Geometry check sheet. Reference: the model listing, model coordinates, mm. A direction names the side the tool comes from. Round coordinates to 2 decimals unless told otherwise and drop trailing zeros. Write each loop counter-clockwise with the first axis right and the second up, starting at its lowest first coordinate (ties: lowest second). Pieces come first, ordered by that corner, then holes.
Item 1: Cross-section at C-C (y = 18). Enter the section's corners in (x, z), then the cut area to 3 significant figures.
Item 2: Access from +Z, -Z, +X, -X, +Y, -Y to the whole of each face (thin tool, end or side, straight path). Record for faces 5 (the face through (7.612, 15, -63)), 6 (the face through (20, 6, -109)), 7 (the face through (47.99, 6.55, -21.06)), 8 (the face through (34.094, 10, -63)).
Item 3: Cross-section at A-A (x = 18). Enter the section's corners in (y, z).
Item 4: Cross-section at B-B (z = -104). Enter the section's corners in (x, y).
Item 5: Depth check by flat-ended pin: P1, Ø6, axis at x = 30.5, z = -69, coming from the +Y side; P2, Ø10, axis at y = 15, z = -103, coming from the +X side; P3, Ø1.5, axis at x = 34, y = 8.5, coming from the +Z side; P4, Ø1.7, axis at y = 10, z = -20, coming from the -X side. Enter the tip coordinate at first touch or a pass-through.
Item 6: Draft check along Z on faces 1 (the face through (40, 10, -59)), 2 (the face through (-2.96, 7.24, -98.07)), 3 (the face through (4.34, 9.86, -54.587)), 4 (the face through (48, 10, -30)). Enter one of: pulls with the +Z half, pulls with the -Z half, needs draft (parallel to the pull), parting line crosses it, or undercut.
Item 7: Cross-section at D-D (x = 36.5). Enter the section's corners in (y, z).
Item 8: Scan lines: probe 1 along Z at (x, y) = (26.5, 14.75); probe 2 along Y at (x, z) = (15, -109); probe 3 along X at (y, z) = (14, -20.5). Record each from-to range of solid material in increasing order.
from build123d import *

# Parameters (mm, degrees)
AUFSATZ_LINEAR_AUSTRAGEN1_DEPTH      = 20
SCHNITT_LINEAR_AUSTRAGEN1_DEPTH      = 53.24
SKIZZE3_R                            = 3.1
SCHNITT_LINEAR_AUSTRAGEN2_DEPTH      = 53.24
SCHNITT_LINEAR_AUSTRAGEN3_DEPTH      = 2
SKIZZE5_R                            = 0.75
SCHNITT_LINEAR_AUSTRAGEN4_DEPTH      = 2
AUFSATZ_LINEAR_AUSTRAGEN2_DEPTH      = 20
SKIZZE7_W                            = 7.611739691
SKIZZE7_H                            = 51.890970688
AUFSATZ_LINEAR_AUSTRAGEN3_DEPTH      = 20
SKIZZE8_W                            = 11.248625368
SKIZZE8_H                            = 20
AUFSATZ_LINEAR_AUSTRAGEN4_DEPTH      = 26.48
SCHNITT_LINEAR_AUSTRAGEN5_DEPTH      = 26.48
SCHNITT_LINEAR_AUSTRAGEN6_DEPTH      = 6
SCHNITT_LINEAR_AUSTRAGEN6_DEPTH_BACK = 26.48
SKIZZE10_R                           = 1.75
SKIZZE11_R                           = 3
AUFSATZ_LINEAR_AUSTRAGEN5_DEPTH      = 6


with BuildPart() as part:
    # Skizze1 → Aufsatz-Linear austragen1 (new body)
    with BuildSketch(Plane(origin=(0, 0, 0), x_dir=(1, 0, 0), z_dir=(0, 1, 0))):
        with BuildLine():
            Line((0, 59), (0, 0))
            Line((0, 0), (3, 0))
            Line((3, 0), (3, 51.3))
            ThreePointArc((3, 51.3), (4.376598128, 54.623401872), (7.7, 56))
            Line((7.7, 56), (42.3, 56))
            ThreePointArc((42.3, 56), (45.623401872, 54.623401872), (47, 51.3))
            Line((47, 51.3), (47, 0))
            Line((47, 0), (50, 0))
            Line((50, 0), (50, 54.3))
            ThreePointArc((50, 54.3), (48.623401872, 57.623401872), (45.3, 59))
            Line((45.3, 59), (0, 59))
        make_face()
    extrude(amount=AUFSATZ_LINEAR_AUSTRAGEN1_DEPTH)

    # Skizze2 → Schnitt-Linear austragen1 (cut)
    with BuildSketch(Plane(origin=(50, 0, 0), x_dir=(0, 0, -1), z_dir=(1, 0, 0))):
        with BuildLine():
            ThreePointArc((0, 10), (2.928932188, 17.071067812), (10, 20))
            Line((10, 20), (0, 20))
            Line((0, 20), (0, 10))
        make_face()
        with BuildLine():
            ThreePointArc((10, 0), (2.928932188, 2.928932188), (0, 10))
            Line((0, 10), (0, 0))
            Line((0, 0), (10, 0))
        make_face()
    extrude(amount=-SCHNITT_LINEAR_AUSTRAGEN1_DEPTH, mode=Mode.SUBTRACT)

    # Skizze3 → Schnitt-Linear austragen2 (cut)
    with BuildSketch(Plane(origin=(50, 0, 0), x_dir=(0, 0, -1), z_dir=(1, 0, 0))):
        with Locations((10, 10)):
            Circle(SKIZZE3_R)
    extrude(amount=-SCHNITT_LINEAR_AUSTRAGEN2_DEPTH, mode=Mode.SUBTRACT)

    # Skizze4 → Schnitt-Linear austragen3 (cut)
    with BuildSketch(Plane.ZY.offset(-47)):
        with BuildLine():
            Line((-27.5, 12.5), (-14.807252725, 14.374965285))
            ThreePointArc((-14.807252725, 14.374965285), (-3.5, 10), (-14.807252725, 5.625034715))
            Line((-14.807252725, 5.625034715), (-27.5, 7.5))
            ThreePointArc((-27.5, 7.5), (-30, 10), (-27.5, 12.5))
        make_face()
    extrude(amount=-SCHNITT_LINEAR_AUSTRAGEN3_DEPTH, mode=Mode.SUBTRACT)

    # Skizze5 → Schnitt-Linear austragen4 (cut)
    with BuildSketch(Plane.ZY.offset(-49)):
        with Locations((-25.995480757, 10)):
            Circle(SKIZZE5_R)
        with Locations((-22.995480757, 10)):
            Circle(SKIZZE5_R)
        with Locations((-19.995480757, 10)):
            Circle(SKIZZE5_R)
        with Locations((-16.995480757, 10)):
            Circle(SKIZZE5_R)
    extrude(amount=-SCHNITT_LINEAR_AUSTRAGEN4_DEPTH, mode=Mode.SUBTRACT)

    # Skizze6 → Aufsatz-Linear austragen2 (add)
    with BuildSketch(Plane.XZ):
        Polygon((34.094038703, -59.256850744), (34.094038703, -67.256850744), (0, -67.256850744), (0, -59.256850744), (0, -57.894447073), (34.094038703, -57.894447073), align=None)
    extrude(amount=-AUFSATZ_LINEAR_AUSTRAGEN2_DEPTH)

    # Skizze7 → Aufsatz-Linear austragen3 (add)
    with BuildSketch(Plane.XZ):
        with Locations((3.805869846, -93.202336088)):
            Rectangle(SKIZZE7_W, SKIZZE7_H)
    extrude(amount=-AUFSATZ_LINEAR_AUSTRAGEN3_DEPTH)

    # Skizze8 → Aufsatz-Linear austragen4 (add)
    with BuildSketch(Plane(origin=(7.611739691, 0, 0), x_dir=(0, 0, -1), z_dir=(1, 0, 0))):
        with Locations((113.523508748, 10)):
            Rectangle(SKIZZE8_W, SKIZZE8_H)
    extrude(amount=AUFSATZ_LINEAR_AUSTRAGEN4_DEPTH)

    # Skizze9 → Schnitt-Linear austragen5 (cut)
    with BuildSketch(Plane(origin=(0, 0, -119.147821432), x_dir=(-1, 0, 0), z_dir=(0, 0, -1))):
        with BuildLine():
            Line((-9.3, 14), (-29.794038703, 14))
            ThreePointArc((-29.794038703, 14), (-31.066830909, 13.472792206), (-31.594038703, 12.2))
            Line((-31.594038703, 12.2), (-31.594038703, 7.8))
            ThreePointArc((-31.594038703, 7.8), (-31.066830909, 6.527207794), (-29.794038703, 6))
            Line((-29.794038703, 6), (-9.3, 6))
            ThreePointArc((-9.3, 6), (-8.027207794, 6.527207794), (-7.5, 7.8))
            Line((-7.5, 7.8), (-7.5, 12.2))
            ThreePointArc((-7.5, 12.2), (-8.027207794, 13.472792206), (-9.3, 14))
        make_face()
    extrude(amount=-SCHNITT_LINEAR_AUSTRAGEN5_DEPTH, mode=Mode.SUBTRACT)

    # Skizze10 → Schnitt-Linear austragen6 (cut, two sides: drawn at the far end of the back side and taken through both)
    with BuildSketch(Plane(origin=(34.091739691, 0, 0), x_dir=(0, 0, -1), z_dir=(1, 0, 0)).offset(-SCHNITT_LINEAR_AUSTRAGEN6_DEPTH_BACK)):
        with Locations((62.806850744, 14.75)):
            Circle(SKIZZE10_R)
        with Locations((62.806850744, 5.05)):
            Circle(SKIZZE10_R)
        with Locations(Location((112.406850744, 5.05, 0), (0, 0, 180))):
            Circle(SKIZZE10_R)
        with Locations(Location((112.406850744, 14.75, 0), (0, 0, 180))):
            Circle(SKIZZE10_R)
    extrude(amount=SCHNITT_LINEAR_AUSTRAGEN6_DEPTH + SCHNITT_LINEAR_AUSTRAGEN6_DEPTH_BACK, mode=Mode.SUBTRACT)

    # Skizze11 → Aufsatz-Linear austragen5 (add)
    with BuildSketch(Plane.ZY):
        with Locations((-99.456850744, 9.9)):
            Circle(SKIZZE11_R)
    extrude(amount=AUFSATZ_LINEAR_AUSTRAGEN5_DEPTH)


solid = part.part
Resolved:
1. outline: (0, -119.15) - (34.09, -119.15) - (34.09, -107.9) - (7.61, -107.9) - (7.61, -67.26) - (34.09, -67.26) - (34.09, -59) - (45.3, -59) arc R4.7 ccw to (50, -54.3) - (50, -4) - (47, -4) - (47, -51.3) arc R4.7 cw to (42.3, -56) - (7.7, -56) arc R4.7 cw to (3, -51.3) - (3, -4) - (0, -4) - close
1. area: 1,440 mm2
2. face 5: +X
2. face 6: -Z
2. face 7: none
2. face 8: -Z, +X, +Y, -Y
3. outline: (0, -119.15) - (6, -119.15) - (6, -113.88) arc R1.75 cw (long way) to (6, -110.94) - (6, -107.9) - (0, -107.9) - close; (0, -67.26) - (20, -67.26) - (20, -56) - (0, -56) - close; (14, -119.15) - (20, -119.15) - (20, -107.9) - (14, -107.9) - (14, -110.83) arc R1.75 cw (long way) to (14, -113.99) - close; hole circle Ø3.5 at (5.05, -62.81); hole circle Ø3.5 at (14.75, -62.81)
4. outline: (0, 0) - (7.61, 0) - (7.61, 7.18) arc R1.8 cw to (7.5, 7.8) - (7.5, 12.2) arc R1.8 cw to (7.61, 12.82) - (7.61, 20) - (0, 20) - close
5. P1: stops at y = 20
5. P2: stops at x = 34.09
5. P3: stops at z = -56
5. P4: stops at x = 0
6. face 1: pulls with the -Z half
6. face 2: parting line crosses it
6. face 3: pulls with the +Z half
6. face 4: undercut
7. outline: (0, -59) - (20, -59) - (20, -56) - (0, -56) - close
8. probe 1: z = -119.15 to -114.16, -110.66 to -107.9, -67.26 to -64.56, -61.06 to -56
8. probe 2: y = 0 to 6, 14 to 20
8. probe 3: x = 0 to 3, 47 to 50
